For this review, use the dimensioned drawing (mm, ordinates from the lowest corner) and the shaded views. Give positions to 0.01 mm unless a question says otherwise; leave off trailing zeros. Write each loop counter-clockwise with the first axis right and the second up, starting at its lowest first coordinate (ties: lowest second). Pieces come first, ordered by that corner, then holes. Notation, with made-up numbers: M 19.25,61 L 51.25,61 A34 ccw 51.25,97 Z; hole C 4.25,39 d6. An arc over 180 degrees is marked long. One line per item, written item: value. Start each with the question number.
Item 1: To check wall thickness, follow probe 1 along X at (y, z) = (3.35, 4.5) (1 decimal); probe 2 along X at (y, z) = (2.15, 6) (1 decimal); probe 3 along Z at (x, y) = (4, 1.5) (1 decimal). State the ranges of each line that lie inside material, in increasing order.
Item 2: Mouldability with a two-part tool opening along X and no side actions: class the marked faces 1, 2, 3 and 4 as released by +X, released by -X, zero draft, split by the parting line, or undercut.
Item 3: Consider section D-D, the plane x = 1. Write out the cut boundary in (y, z), and give its area (3 significant figures).
Item 4: Consider section C-C, the plane y = 3.7. Write out the cut boundary in (x, z) (1 decimal).
Item 5: Consider section B-B, the plane z = 7. Write out the cut boundary in (x, y).
Item 6: Clearance check with a flat-ended pin moving along its axis: pin 1 Ø2 at (x, z) = (9, 4) entering from -Y. State where the tip first meets the part, or that it passes through.
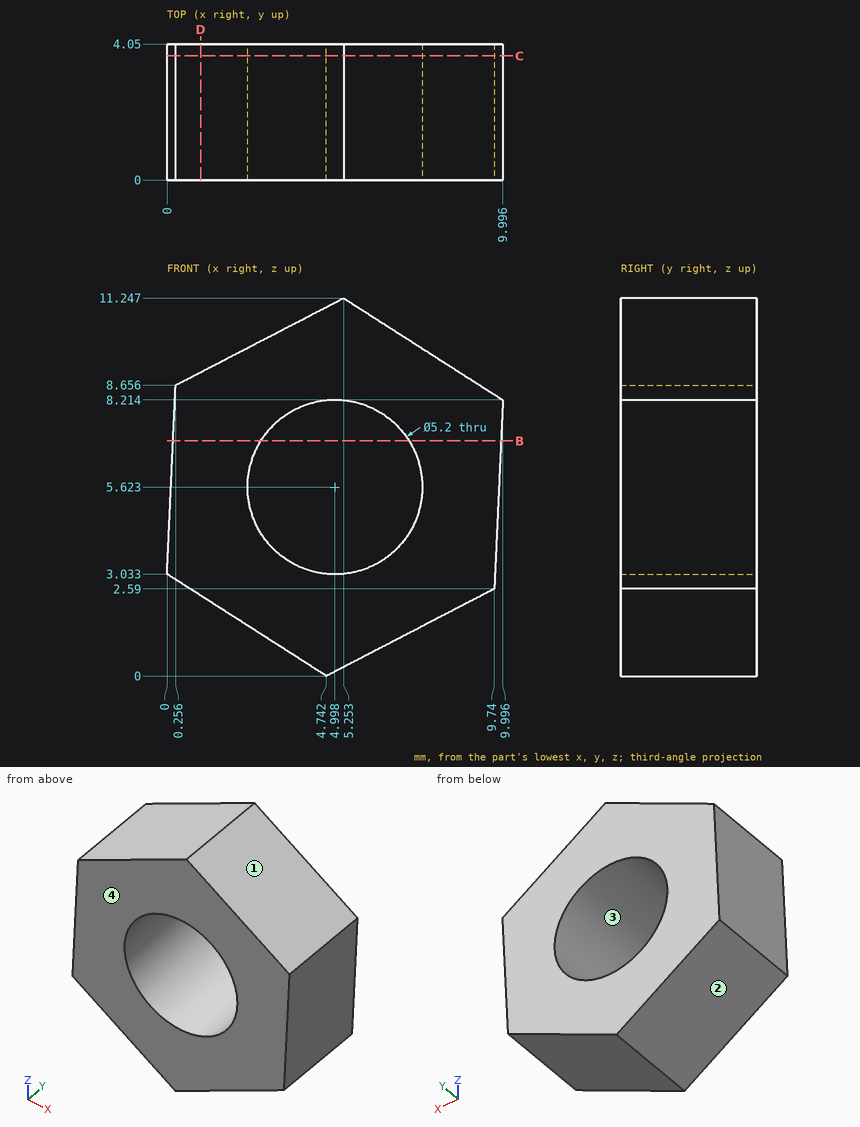
Model answer:
1. probe 1: x = 0.1 to 2.7, 7.3 to 9.8
1. probe 2: x = 0.1 to 2.4, 7.6 to 9.9
1. probe 3: z = 0.5 to 3.2, 8 to 10.6
2. face 1: released by +X
2. face 2: released by -X
2. face 3: undercut
2. face 4: zero draft
3. outline: M 0,2.39 L 4.05,2.39 L 4.05,9.04 L 0,9.04 Z
3. area: 26.9 mm2
4. outline: M 0,3 L 4.7,0 L 9.7,2.6 L 10,8.2 L 5.3,11.2 L 0.3,8.7 Z; hole C 5,5.6 d5.2
5. outline: M 0.18,0 L 2.79,0 L 2.79,4.05 L 0.18,4.05 Z; M 7.2,0 L 9.94,0 L 9.94,4.05 L 7.2,4.05 Z
6. pin 1: stops at y = 0
